For this review, take the finished solid that the model builds, in its own axes (mm). Round coordinates to 2 decimals unless told otherwise and drop trailing zeros. Order: outer loops, then holes, each group sorted by start corner. A loop starts at its lowest first (then second) coordinate and runs counter-clockwise, first axis right, second up. Notation, with made-up numbers: M 5.5,15.25 L 34.5,15.25 A12 ccw 34.5,21.25 Z; hole C 61,39.25 d4. An arc over 180 degrees is marked long. Put each result on its own line as item: value.
from build123d import *

# Parameters (mm, degrees)
SKETCH1_W           = 965.2
SKETCH1_H           = 508
BOSS_EXTRUDE1_DEPTH = 190.5
SKETCH2_W           = 38.1
SKETCH2_H           = 19.05
BOSS_EXTRUDE3_DEPTH = 38.1
SKETCH3_R           = 12.7
CUT_EXTRUDE1_DEPTH  = 19.05
CUT_EXTRUDE2_REACH  = 510
SKETCH2_4_R         = 12.7


with BuildPart() as part:
    # Sketch1 → Boss-Extrude1 (new body)
    with BuildSketch(Plane(origin=(0, 0, 0), x_dir=(1, 0, 0), z_dir=(0, 1, 0))):
        Rectangle(SKETCH1_W, SKETCH1_H)
    extrude(amount=BOSS_EXTRUDE1_DEPTH)

    # Sketch2 → Boss-Extrude3 (add)
    with BuildSketch(Plane.XY.offset(254)):
        with Locations((254, 63.5)):
            Rectangle(SKETCH2_W, SKETCH2_H)
    boss_extrude3 = extrude(amount=BOSS_EXTRUDE3_DEPTH)

    # Sketch3 → Cut-Extrude1 (cut)
    with BuildSketch(Plane(origin=(0, 73.025, 0), x_dir=(1, 0, 0), z_dir=(0, 1, 0))):
        with Locations((254, -273.05)):
            Circle(SKETCH3_R)
    cut_extrude1 = extrude(amount=-CUT_EXTRUDE1_DEPTH, mode=Mode.SUBTRACT)

    # Sketch2_4 → Cut-Extrude2 (cut, up to next)
    with BuildSketch(Plane.XY.offset(254), mode=Mode.PRIVATE) as cut_extrude2_sk1:
        with Locations((-254, 25.4)):
            Circle(SKETCH2_4_R)
    cut_extrude2_tool1 = extrude(cut_extrude2_sk1.sketch, amount=-CUT_EXTRUDE2_REACH, mode=Mode.PRIVATE) & part.part
    add(cut_extrude2_tool1.solids().sort_by_distance((-254, 25.4, 254))[0], mode=Mode.SUBTRACT)

    # Mirror2: Boss-Extrude3, Cut-Extrude1 across plane
    add(boss_extrude3.mirror(Plane.XY))
    add(cut_extrude1.mirror(Plane.XY), mode=Mode.SUBTRACT)


solid = part.part
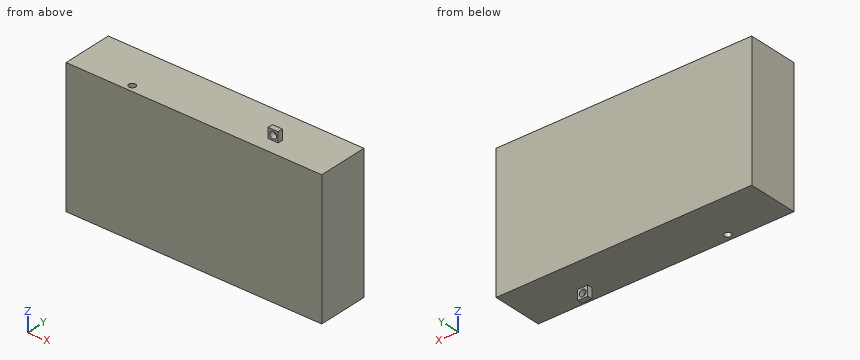
(1) Add section A-A on x = -254. Give the boundary of the cut face in (y, z), then the cut area to 3 significant figures.
A:
outline: M 0,-254 L 12.7,-254 L 12.7,254 L 0,254 Z; M 38.1,-254 L 190.5,-254 L 190.5,254 L 38.1,254 Z
area: 83,900 mm2
(2) Add section C-C on z = 273.05. Give the boundary of the cut face in (x, y) (3 decimals).
A:
outline: M 234.95,53.975 L 241.3,53.975 L 241.3,73.025 L 234.95,73.025 Z; M 266.7,53.975 L 273.05,53.975 L 273.05,73.025 L 266.7,73.025 Z
(3) Add section B-B on x = 254. Give the boundary of the cut face in (y, z) (3 decimals), then the cut area to 3 significant figures.
A:
outline: M 0,-254 L 53.975,-254 L 53.975,-260.35 L 73.025,-260.35 L 73.025,-254 L 190.5,-254 L 190.5,254 L 73.025,254 L 73.025,260.35 L 53.975,260.35 L 53.975,254 L 0,254 Z; M 53.975,-292.1 L 73.025,-292.1 L 73.025,-285.75 L 53.975,-285.75 Z; M 53.975,285.75 L 73.025,285.75 L 73.025,292.1 L 53.975,292.1 Z
area: 97,300 mm2
(4) Add section D-D on y = 101.5. Give the boundary of the cut face in (x, z), then the cut area to 3 significant figures.
A:
outline: M -482.6,-254 L 482.6,-254 L 482.6,254 L -482.6,254 Z
area: 490,000 mm2
(5) Insertion check: pin 1 Ø9.5 at (y, z) = (66, -276.5) entering from -X; pin 2 Ø2 at (x, y) = (110, 28.5) entering from +Z; pin 3 Ø5.5 at (y, z) = (60, 276.5) entering from +X. Each pin has a flat end and moves straight along its axis. Give the tip position at first contact, or say it passes through.
A:
pin 1: stops at x = 234.95
pin 2: stops at z = 254
pin 3: stops at x = 273.05
(6) To check wall thickness, follow L1, parallel to Z at x = 254, y = 65.25; L2, parallel to Y at x = -254, z = 26; L3, parallel to X at y = 64, z = -273.05. State the ranges of each line that lie inside material, in increasing order.
A:
L1: z = -292.1 to -285.75, -260.35 to 260.35, 285.75 to 292.1
L2: y = 0 to 12.7, 38.1 to 190.5
L3: x = 234.95 to 241.3, 266.7 to 273.05
